For this review, take the finished solid that the model builds, in its own axes (mm). A direction names the side the tool comes from. Round coordinates to 2 decimals unless told otherwise and drop trailing zeros. Write each loop counter-clockwise with the first axis right and the second up, starting at its lowest first coordinate (ties: lowest second). Pieces come first, ordered by that corner, then holes. Notation, with made-up numbers: M -6,-21.75 L 8,-21.75 A27 ccw 8,-2.75 Z; hole C 85.5,45.5 d10. An arc over 180 degrees is marked long. Use one line per item in the form item = value. Start each with the question number.
Item 1: For line 1 (X direction, y = 40, z = -8); line 2 (X direction, y = 39.5, z = -52.5), list the stretches that pass through material, from the lowest coordinate up. Write a range as [from, to].
Item 2: Add section A-A (x = 30). State the section outline as (y, z) points, and give its area (3 significant figures).
Item 3: Draft analysis for pull direction Y (two halves, no side actions). For faces 5 (the flat face through (48.26, 26, -6)), 6 (the flat face through (24, 1, -64.008)), 7 (the flat face through (26, 52.07, -38)), state which applies: released by +Y, released by -Y, zero draft, split by the parting line, or undercut.
Item 4: Add section C-C (z = -70). State the section outline as (x, y) points, and give its area (3 significant figures).
Item 5: Add section D-D (x = 5). State the section outline as (y, z) points.
Item 6: For faces 1 (the cylindrical face through (8.26, 8.16, -38.46)), 2 (the flat face through (49.53, 26, -70)), 3 (the flat face through (3.81, 26, -6)), 4 (the flat face through (48.26, 26, -70)), list the 3-axis set-ups (+Z, -Z, +X, -X, +Y, -Y) from which the entire face can be reached by the end or side of a thin tool; tool diameter is ignored.
Item 7: For P1, Ø8, axis at x = 39, z = -36, coming from the -Y side; P2, Ø6, axis at y = 27.5, z = -69.5, coming from the +X side; P3, Ø10, axis at x = 30.5, z = -73, coming from the -Y side; P4, Ø22, axis at x = 21.5, y = 22, coming from the -Z side, all flat-tipped, find the tip position at first contact; note any pin that passes through.
from build123d import *

# Parameters (mm, degrees)
SKETCH1_W           = 52.07
SKETCH1_H           = 52.07
BOSS_EXTRUDE1_DEPTH = 76.2
SKETCH2_W           = 39.37
SKETCH2_H           = 39.37
CUT_EXTRUDE1_DEPTH  = 106.967022229
SKETCH3_W           = 52.07
SKETCH3_H           = 52.07
SKETCH3_W_2         = 46.99
SKETCH3_H_2         = 46.99
SKETCH3_W_3         = 44.45
SKETCH3_H_3         = 44.45
SKETCH3_W_4         = 39.37
SKETCH3_H_4         = 39.37
CUT_EXTRUDE2_DEPTH  = 12.192
FILLET1_R           = 6.35


with BuildPart() as part:
    # Sketch1 → Boss-Extrude1 (new body)
    with BuildSketch(Plane.XY):
        with Locations((26.035, 26.035)):
            Rectangle(SKETCH1_W, SKETCH1_H)
    extrude(amount=-BOSS_EXTRUDE1_DEPTH)

    # Sketch2 → Cut-Extrude1 (cut, through all)
    with BuildSketch(Plane.XY):
        with Locations((26.035, 26.035)):
            Rectangle(SKETCH2_W, SKETCH2_H)
    extrude(amount=-CUT_EXTRUDE1_DEPTH, mode=Mode.SUBTRACT)

    # Sketch3 → Cut-Extrude2 (cut)
    # profile 1 of 2: a face of its own
    with BuildSketch(Plane.XY):
        with Locations((26.035, 26.035)):
            Rectangle(SKETCH3_W, SKETCH3_H)
        with Locations((26.035, 26.035)):
            Rectangle(SKETCH3_W_2, SKETCH3_H_2, mode=Mode.SUBTRACT)
    # profile 2 of 2: a face of its own
    with BuildSketch(Plane.XY):
        with Locations((26.035, 26.035)):
            Rectangle(SKETCH3_W_3, SKETCH3_H_3)
        with Locations((26.035, 26.035)):
            Rectangle(SKETCH3_W_4, SKETCH3_H_4, mode=Mode.SUBTRACT)
    cut_extrude2 = extrude(amount=-CUT_EXTRUDE2_DEPTH, mode=Mode.SUBTRACT)

    # Mirror1: Cut-Extrude2 across plane
    add(cut_extrude2.mirror(Plane(origin=(0, 0, -38.1), x_dir=(1, 0, 0), z_dir=(0, 0, -1))), mode=Mode.SUBTRACT)

    # Fillet1
    fillet1_edges = [part.edges().sort_by_distance(p)[0] for p in [
        (45.72, 6.35, -38.1),
        (6.35, 6.35, -38.1),
        (45.72, 45.72, -38.1),
        (6.35, 45.72, -38.1),
    ]]
    fillet(fillet1_edges, radius=FILLET1_R)


solid = part.part
Calculated:
q1.line_1 = [2.54, 3.81], [48.26, 49.53]
q1.line_2 = [0, 6.35], [45.72, 52.07]
q2.outline = M 0,-64.01 L 2.54,-64.01 L 2.54,-76.2 L 3.81,-76.2 L 3.81,-64.01 L 6.35,-64.01 L 6.35,-12.19 L 3.81,-12.19 L 3.81,0 L 2.54,0 L 2.54,-12.19 L 0,-12.19 Z; M 45.72,-64.01 L 48.26,-64.01 L 48.26,-76.2 L 49.53,-76.2 L 49.53,-64.01 L 52.07,-64.01 L 52.07,-12.19 L 49.53,-12.19 L 49.53,0 L 48.26,0 L 48.26,-12.19 L 45.72,-12.19 Z
q2.area = 720 mm^2
q3.face_5 = undercut
q3.face_6 = zero draft
q3.face_7 = released by +Y
q4.outline = M 2.54,2.54 L 49.53,2.54 L 49.53,49.53 L 2.54,49.53 Z; hole M 3.81,3.81 L 48.26,3.81 L 48.26,48.26 L 3.81,48.26 Z
q4.area = 232 mm^2
q5.outline = M 0,-64.01 L 2.54,-64.01 L 2.54,-76.2 L 3.81,-76.2 L 3.81,-64.01 L 48.26,-64.01 L 48.26,-76.2 L 49.53,-76.2 L 49.53,-64.01 L 52.07,-64.01 L 52.07,-12.19 L 49.53,-12.19 L 49.53,0 L 48.26,0 L 48.26,-12.19 L 3.81,-12.19 L 3.81,0 L 2.54,0 L 2.54,-12.19 L 0,-12.19 Z
q6.face_1 = +Z, -Z
q6.face_2 = -Z, +X, +Y, -Y
q6.face_3 = +Z
q6.face_4 = -Z
q7.P1 = 0
q7.P2 = 49.53
q7.P3 = 2.54
q7.P4 = through
